Source: CAD feature listing. Evaluate the final solid. Frame: model axes, mm. Face numbers are marked on the shaded views. A direction names the side the tool comes from. Round coordinates to 2 decimals unless told otherwise and drop trailing zeros. Loops run counter-clockwise (first coordinate to the right, second up) from the corner with the lowest first, then second, coordinate; pieces in that order, holes last.
Item 1: Pull-direction query (X, two-part tool) for the marked faces 1, 2 and 3; classes: released by +X, released by -X, zero draft, split by the parting line, or undercut.
Item 2: Section query C-C on x = -3.5. Return loops of the section in (y, z).
Item 3: Section query A-A on z = -7.5. Return loops of the section in (x, y) (1 decimal).
Item 4: First-contact query: P1, Ø8, axis at x = -6, y = 21, coming from the -Z side; P2, Ø1, axis at x = 13.5, z = -7.5, coming from the -Y side; P3, Ø1, axis at y = -25.5, z = 3.5, coming from the +X side; P4, Ø8, axis at y = -24.5, z = -6.5, coming from the -X side. Flat tips, straight axial feed; report the tip coordinate or a pass-through.
Item 5: Ray query, L1, parallel to Z at x = -17.5, y = -3; L2, parallel to Y at x = -8, z = -4.5; L3, parallel to X at y = 9, z = 5.5. Return the intervals inside material, ascending.
Item 6: Section query B-B on x = 8. Return loops of the section in (y, z) (3 decimals).
Item 7: Access query for the marked faces 4, 5 and 6. Directions: +Z, -Z, +X, -X, +Y, -Y. A direction counts if a zero-diameter tool reaches every point of the face in a straight line with its end or side. Return the directions, or none.
Autodesk Inventor part; units mm, degrees
ref_plane "YZ Plane" through (0, 0, 0) normal (1, 0, 0) x (0, 1, 0)
ref_plane "XZ Plane" through (0, 0, 0) normal (0, 1, 0) x (-1, 0, 0)
ref_plane "XY Plane" through (0, 0, 0) normal (0, 0, 1) x (1, 0, 0)
sketch "Boceto1" plane through (0, 0, 0) normal (0, 0, 1) x (1, 0, 0)
  circle A0 centre (0, 0) radius 32.5
  circle A1 centre (0, 0) radius 10
  line L0 (0, -32.5) -> (0, 0) construction
  line L1 (0, -32.5) -> (-9.058, -23.9422)
  line L2 (-9.058, -23.9422) -> (-10.8513, -30.6349)
  dimension "d0" = 65
  dimension "d1" = 20
  dimension "d4" = 15
extrude "Extrusión1" add sketch "Boceto1" along normal blind 12
sketch "Boceto2" plane through (0, 0, 12) normal (0, 0, 1) x (1, 0, 0)
  line L0 (-32.5, 0) -> (0, 0) construction
  line L1 (-32.5, 0) -> (-28.1293, -8)
  line L2 (-28.1293, -8) -> (-31.5, -8)
  circle A0 centre (0, 0) radius 29.2448 construction
  arc A1 (-32.5, 0) -> (-31.5, -8) centre (0, 0) ccw construction
  arc A2 (-32.5, 0) -> (-31.5, -8) centre (0, 0) ccw construction
  circle A3 centre (0, 0) radius 10
  arc A4 (-32.5, 0) -> (-31.5, -8) centre (0, 0) ccw
  dimension "d5" = 8
  dimension "d7" = 8
  dimension "d22" = 20
extrude "Extrusión2" cut sketch "Boceto2" against normal blind 12 contours L1 L2 A4
pattern_circular "Patrón circular1" count 25 over 360 about axis through (0, 0, -10) along (0, 0, 1) of "Extrusión2"
sketch "Boceto3" plane through (0, 0, 0) normal (0, 0, -1) x (-1, 0, 0)
  circle A0 centre (0, 0) radius 17.5
  circle A1 centre (0, 0) radius 10
  dimension "d13" = 35
  dimension "d23" = 20
extrude "Extrusión3" add sketch "Boceto3" along normal blind 12
sketch "Boceto5" plane through (0, 0, -12) normal (0, 0, -1) x (-1, 0, 0)
  circle A0 centre (0, 0) radius 10
  line L0 (11.725, -3.5) -> (8.275, 3.5) construction
  line L1 (8.275, -3.5) -> (11.725, 3.5) construction
  line L2 (9.3675, 3.5) -> (11.725, 3.5)
  line L3 (11.725, -3.5) -> (9.3675, -3.5)
  arc A1 (9.3675, 3.5) -> (9.3675, -3.5) centre (0, 0) ccw
  line L4 (11.725, 3.5) -> (11.725, -3.5)
  dimension "d24" = 3.45
  dimension "d25" = 7
extrude "Extrusión4" cut sketch "Boceto5" against normal blind 24 contours A0 L2 L4 L3
properties part number "Pieza Propia Ensamblaje - Alison"
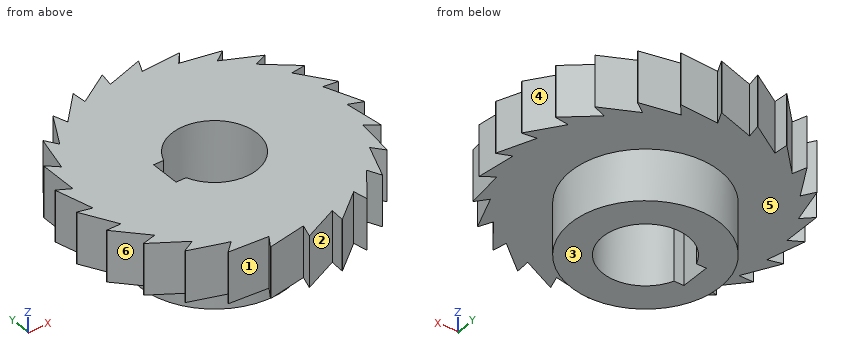
Data:
1. face 1: released by -X
1. face 2: undercut
1. face 3: zero draft
2. outline: (-29.68, 0) - (-17.15, 0) - (-17.15, -12) - (-9.37, -12) - (-9.37, 12) - (-29.68, 12) - close; (9.37, -12) - (17.15, -12) - (17.15, 0) - (31.52, 0) - (31.52, 12) - (9.37, 12) - close
3. outline: circle Ø35 at (0, 0); hole (-11.7, -3.5) - (-9.4, -3.5) arc R10 ccw (long way) to (-9.4, 3.5) - (-11.7, 3.5) - close
4. P1: stops at z = 0
4. P2: stops at y = -11.72
4. P3: stops at x = 20.73
4. P4: passes through
5. L1: z = 0 to 12
5. L2: y = -15.56 to -6, 6 to 15.56
5. L3: x = -28.5 to -4.36, 4.36 to 28.68
6. outline: (-30.353, 0) - (-15.564, 0) - (-15.564, -12) - (-6, -12) - (-6, 12) - (-30.353, 12) - close; (6, -12) - (15.564, -12) - (15.564, 0) - (29.055, 0) - (29.055, 12) - (6, 12) - close
7. face 4: +Z, -Z, +X
7. face 5: -Z
7. face 6: +Z, -Z, -X
